Input: part model. Units: mm. Frame: model coordinates. Face numbers are marked on the shaded views. A direction names the side the tool comes from. Give positions to 0.01 mm unless a question says otherwise; leave off trailing zeros. Loops run counter-clockwise (first coordinate to the right, second up) from the corner with the lowest first, then second, coordinate; pieces in that order, holes last. Notation, with made-up numbers: (-20.5, 27.25) - (2.5, 27.25) arc R14 cw to (2.5, 36.25) - close; hole circle Ø9 at (0, 19). An arc over 180 degrees is marked (long way). Answer as a JSON object with one key per item and string values.
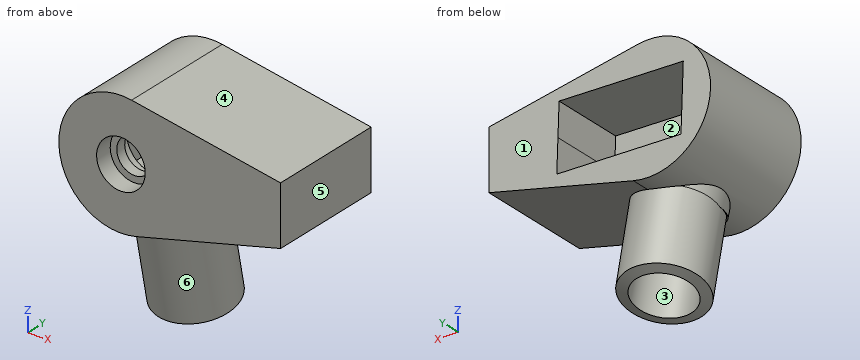
from build123d import *

# Parameters (mm, degrees)
CROQUIS1_R              = 21
SALIENTE_EXTRUIR1_DEPTH = 40
SALIENTE_EXTRUIR2_DEPTH = 40
SALIENTE_EXTRUIR3_REACH = 77.493
CROQUIS3_R              = 13.5
CROQUIS3_R_2            = 10
CROQUIS7_R              = 8.227269221
CROQUIS7_R_2            = 6
CORTAR_EXTRUIR6_DEPTH   = 6
CROQUIS8_R              = 6
CORTAR_EXTRUIR7_DEPTH   = 72.223648425
CORTAR_EXTRUIR8_START   = -25
CORTAR_EXTRUIR8_DEPTH   = 25
CROQUIS12_R             = 9.55
CORTAR_EXTRUIR9_DEPTH   = 5.5


with BuildPart() as part:
    # Croquis1 → Saliente-Extruir1 (new body)
    with BuildSketch(Plane(origin=(0, 0, 0), x_dir=(1, 0, 0), z_dir=(0, 1, 0))):
        with Locations(Location((0, 0, 0), (0, 0, 270))):
            Circle(CROQUIS1_R)
    extrude(amount=SALIENTE_EXTRUIR1_DEPTH)

    # Croquis2 → Saliente-Extruir2 (add)
    with BuildSketch(Plane(origin=(0, 0, 0), x_dir=(1, 0, 0), z_dir=(0, 1, 0))):
        with BuildLine():
            Line((53.975127576, 8.110971331), (53.975127576, -11.889028669))
            Line((53.975127576, -11.889028669), (3.613793412, -20.686722727))
            ThreePointArc((3.613793412, -20.686722727), (20.98607707, -0.764571273), (5.109545014, 20.368911354))
            Line((5.109545014, 20.368911354), (53.975127576, 8.110971331))
        make_face()
    extrude(amount=SALIENTE_EXTRUIR2_DEPTH)

    # Croquis3 → Saliente-Extruir3 (add, up to next)
    with BuildSketch(Plane(origin=(5.109545014, 0, -20.368911354), x_dir=(-0.9699481597219111, 0, -0.24331166731597212), z_dir=(0.2433116673159721, 0, -0.969948159721911)), mode=Mode.PRIVATE) as saliente_extruir3_sk1:
        with Locations((0, 20)):
            Circle(CROQUIS3_R)
        with Locations((0, 20)):
            Circle(CROQUIS3_R_2, mode=Mode.SUBTRACT)
    saliente_extruir3_tool1 = extrude(saliente_extruir3_sk1.sketch, amount=-SALIENTE_EXTRUIR3_REACH, mode=Mode.PRIVATE) - part.part
    add(saliente_extruir3_tool1.solids().sort_by_distance((17.833482, 20, -17.177109))[0])

    # Croquis7 → Cortar-Extruir6 (cut)
    with BuildSketch(Plane.XZ):
        with Locations(Location((0, 0, 0), (0, 0, 270))):
            Circle(CROQUIS7_R)
        with Locations(Location((0, 0, 0), (0, 0, 270))):
            Circle(CROQUIS7_R_2, mode=Mode.SUBTRACT)
    extrude(amount=-CORTAR_EXTRUIR6_DEPTH, mode=Mode.SUBTRACT)

    # Croquis8 → Cortar-Extruir7 (cut, through all)
    with BuildSketch(Plane.XZ):
        with Locations(Location((0, 0, 0), (0, 0, 270))):
            Circle(CROQUIS8_R)
    extrude(amount=-CORTAR_EXTRUIR7_DEPTH, mode=Mode.SUBTRACT)

    # Croquis10 → Cortar-Extruir8 (cut)
    with BuildSketch(Plane(origin=(0, 40, 0), x_dir=(1, 0, 0), z_dir=(0, 1, 0)).offset(CORTAR_EXTRUIR8_START)):
        with BuildLine():
            Line((-5.995438853, 0.23390802), (-11.37823559, 0.424457107))
            Line((-11.37823559, 0.424457107), (-11.767631672, -10.575542893))
            Line((-11.767631672, -10.575542893), (30.232368328, -12.062327932))
            Line((30.232368328, -12.062327932), (30.62176441, -1.062327932))
            Line((30.62176441, -1.062327932), (5.996971268, -0.190619027))
            ThreePointArc((5.996971268, -0.190619027), (-0.212264906, -5.996244125), (-5.995438853, 0.23390802))
        make_face()
        with BuildLine():
            Line((-10.988839509, 11.424457107), (-11.37823559, 0.424457107))
            Line((-11.37823559, 0.424457107), (-5.995438853, 0.23390802))
            ThreePointArc((-5.995438853, 0.23390802), (0.116976243, 5.998859605), (6, 0))
            ThreePointArc((6, 0), (5.999242769, -0.095321543), (5.996971268, -0.190619027))
            Line((5.996971268, -0.190619027), (30.62176441, -1.062327932))
            Line((30.62176441, -1.062327932), (31.011160491, 9.937672068))
            Line((31.011160491, 9.937672068), (-10.988839509, 11.424457107))
        make_face()
    extrude(amount=CORTAR_EXTRUIR8_DEPTH, mode=Mode.SUBTRACT)

    # Croquis12 → Cortar-Extruir9 (cut)
    with BuildSketch(Plane(origin=(0, 15, 0), x_dir=(1, 0, 0), z_dir=(0, 1, 0))):
        with Locations(Location((0, 0, 0), (0, 0, 270))):
            Circle(CROQUIS12_R)
    extrude(amount=-CORTAR_EXTRUIR9_DEPTH, mode=Mode.SUBTRACT)

    # Croquis4 → Revolución2 (revolve)
    with BuildSketch(Plane(origin=(5.1, 0, 0), x_dir=(0, 0, -1), z_dir=(1, 0, 0))):
        Polygon((23.468699932, 10.900780306), (51.668699932, 16.900780306), (51.668699932, 13.400780306), (16.629031587, 5.945531722), (16.629031587, 9.445531722), align=None)
    revolve(axis=Axis((5.1, 20.900780306, -23.468699932), (0, 0.20810764446485977, -0.9781059289848353)))


solid = part.part
Item 1: Material intervals for line 1 (X direction, y = 2.8, z = 0); line 2 (Z direction, x = 15.5, y = 24); line 3 (X direction, y = 8.5, z = 0), sorted ascending. Write a range as [from, to].
Geometry check:
{"line 1": "x = [-21, -8.23], [8.23, 53.98]", "line 2": "z = [-49.96, -10.49], [11.54, 18.61]", "line 3": "x = [-21, -6], [6, 53.98]"}
Item 2: Mould query, pull axis Z, two halves, no side actions, for the marked faces 3, 4, 5 and 6. Classes: released by +Z, released by -Z, zero draft, split by the parting line, or undercut.
Geometry check:
{"face 3": "undercut", "face 4": "released by +Z", "face 5": "zero draft", "face 6": "undercut"}
Item 3: Access query for the marked faces 1 and 2. Directions: +Z, -Z, +X, -X, +Y, -Y. A direction counts if a zero-diameter tool reaches every point of the face in a straight line with its end or side. Return the directions, or none.
Geometry check:
{"face 1": "+Z, -Z, +X, -X, +Y", "face 2": "+Y"}
Item 4: Cut plane B-B (x = 34.5). Return loops of the section in (y, z), then the cut area to 3 significant figures.
Geometry check:
{"outline": "(0, -13) - (40, -13) - (40, 15.29) - (0, 15.29) - close", "area": "1,130 mm2"}
Item 5: Contact query for flat-ended pins moving along their axis: P1, Ø5, axis at x = -4, z = 2, coming from the -Y side; P2, Ø10, axis at y = 16.5, z = -35, coming from the -X side; P3, Ø8, axis at x = 21, z = -27.5, coming from the +Y side. Output: stop coordinate, or through.
Geometry check:
{"P1": "stops at y = 6", "P2": "stops at x = -7.99", "P3": "stops at y = 27.65"}
Item 6: Cut plane A-A (y = 3). Return loops of the section in (x, z), then the cut area to 3 significant figures.
Geometry check:
{"outline": "(3.61, 20.69) arc R21 ccw (long way) to (5.11, -20.37) - (53.98, -8.11) - (53.98, 11.89) - close; hole circle Ø16.45 at (0, 0)", "area": "2,180 mm2"}
